from build123d import *

# Parameters (mm, degrees)
F1_DEPTH = 38.1
F3_DEPTH = 38.101
F4_R     = 1
F6_DEPTH = 38.1
F7_R     = 1
F8_R     = 1


with BuildPart() as f1:
    # F0 (on Top) → F1 (new body)
    with BuildSketch(Plane.XY):
        Polygon((21.9970452561, 0), (0, 38.1), (-21.9970452561, 0), align=None)
    extrude(amount=F1_DEPTH)

    # F2 (on face) → F3 (cut, through all)
    with BuildSketch(Plane.XY.offset(38.1)):
        Polygon((-0.1427694591, 30.6260475565), (-5, 29.4397459622), (-16.9970452561, 8.6602540378), (-15.595797303, 3.8606182002), align=None)
    extrude(amount=-F3_DEPTH, mode=Mode.SUBTRACT)

    # F4
    f4_edges = [f1.edges().sort_by_distance(p)[0] for p in [
        (-5, 29.439746, 19.05),
        (-16.997045, 8.660254, 19.05),
    ]]
    fillet(f4_edges, radius=F4_R)

    # F5 (on face) → F6 (join, through all)
    with BuildSketch(Plane.XY.offset(38.1)):
        Polygon((7.6392122053, 33.5131891134), (5.05, 29.3531434218), (16.9470452561, 8.7468565782), (21.8443566086, 8.909157278), align=None)
    extrude(amount=-F6_DEPTH)

    # F7
    f7_edges = [f1.edges().sort_by_distance(p)[0] for p in [
        (7.639212, 33.513189, 19.05),
        (21.844357, 8.909157, 19.05),
    ]]
    fillet(f7_edges, radius=F7_R)

    # F8
    f8_edges = [f1.edges().sort_by_distance(p)[0] for p in [
        (0, 38.1, 19.05),
        (-21.997045, 0, 19.05),
        (21.997045, 0, 19.05),
    ]]
    fillet(f8_edges, radius=F8_R)


solid = f1.part
Model file for the job. Use its own axes, mm. A direction names the side the tool comes from. Give positions to 0.01 mm unless a question says otherwise; leave off trailing zeros. Write each loop counter-clockwise with the first axis right and the second up, starting at its lowest first coordinate (ties: lowest second). Pieces come first, ordered by that corner, then holes. Notation, with made-up numbers: (68, 12) -> (108, 12) arc R29 ccw to (108, 45) -> close; hole circle Ø10 at (19.25, 29.5). An arc over 180 degrees is marked (long way). Write item = value, one per line.
(1) Mould opens along X. For faces 4 (the face through (5.916, 30.744, 19.317)), 5 (the face through (-21.124, 0.487, 19.317)), 6 (the face through (4, 15, 0)) say: released by +X, released by -X, zero draft, split by the parting line, or undercut.
Determined:
face_4 = undercut
face_5 = released by -X
face_6 = zero draft
(2) Slice it at C-C, the plane x = 6. Give the cut face in (y, z).
Determined:
outline = (0, 0) -> (30.88, 0) -> (30.88, 38.1) -> (0, 38.1) -> close
(3) Slice it at B-B, the plane y = 15. Give the cut face in (x, z).
Determined:
outline = (-9.16, 0) -> (18.33, 0) -> (18.33, 38.1) -> (-9.16, 38.1) -> close
(4) Tool access for faces 1 (the face through (3, 32.9, 18.8)), 2 (the face through (0, 0, 19)), 3 (the face through (19.07, 5.07, 18.78)): list every direction of +Z, -Z, +X, -X, +Y, -Y with a clear straight run to the whole face (end or side of a thin tool).
Determined:
face_1 = +Z, -Z, +Y
face_2 = +Z, -Z, +X, -X, -Y
face_3 = +Z, -Z, +X
(5) Probe line 1 along X through (y, z) = (3, 24.5) (3 decimals); line 2 along X through (y, z) = (32, 19); line 3 along X through (y, z) = (5, 32). List the from-to ranges inside material, lowest first.
Determined:
line_1 = -20.265 to 20.265
line_2 = -3.52 to 3.52, 6.7 to 8.51
line_3 = -19.11 to -15.93, -14.94 to 19.11
(6) Slice it at A-A, the plane z = 30.5. Give the cut face in (x, y) (3 decimals), then the cut area to 3 significant figures.
Determined:
outline = (-21.131, 1.5) arc R1 ccw to (-20.265, 0) -> (20.265, 0) arc R1 ccw to (21.131, 1.5) -> (16.947, 8.747) -> (20.178, 8.854) arc R1 ccw to (21.011, 10.353) -> (8.473, 32.069) arc R1 ccw to (6.758, 32.097) -> (5.05, 29.353) -> (0.866, 36.6) arc R1 ccw to (-0.866, 36.6) -> (-3.83, 31.466) arc R1 ccw to (-2.727, 29.995) -> (-0.143, 30.626) -> (-15.596, 3.861) -> (-16.341, 6.414) arc R1 ccw to (-18.167, 6.634) -> close
area = 846 mm2
(7) Flat gauge pins, fed straight in: P1, Ø1.5, axis at y = 27.5, z = 9.5, coming from the +X side; P2, Ø8, axis at x = 16.5, z = 12, coming from the +Y side; P3, Ø6, axis at y = 32, z = 32, coming from the -X side. Where does each tip first touch, or does it go through?
Determined:
P1 = 11.54
P2 = 25.09
P3 = -3.96
